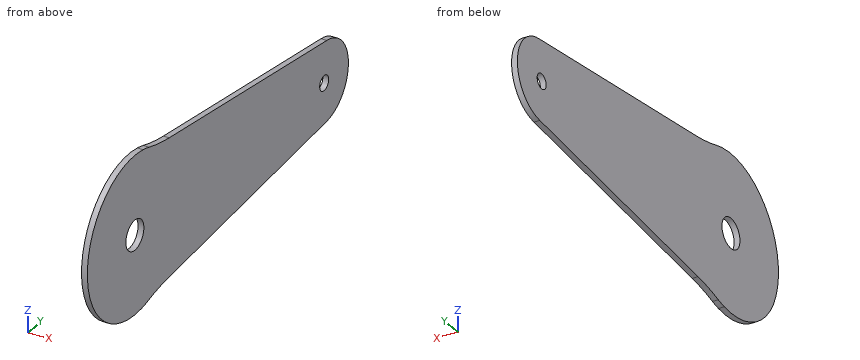
from build123d import *

# Parameters (mm, degrees)
SKETCH_2_R      = 3.85
SKETCH_2_R_2    = 1.925
EXTRUDE_1_DEPTH = 1.5


with BuildPart() as part:
    # 草圖2 → 填料-伸長1 (new body)
    with BuildSketch(Plane(origin=(0, 0, 0), x_dir=(0, 0, -1), z_dir=(1, 0, 0))):
        with BuildLine():
            Line((18.012072511, -21.441606673), (11.718522882, 46.276737912))
            ThreePointArc((11.718522882, 46.276737912), (1.55399875, 55.843411078), (-8.930005845, 46.627965677))
            Line((-8.930005845, 46.627965677), (-17.523002046, -20.837161438))
            ThreePointArc((-17.523002046, -20.837161438), (-18.27264724, -25.183298229), (-19.402359762, -29.446468708))
            ThreePointArc((-19.402359762, -29.446468708), (-19.752456192, -30.70663404), (-20.020797275, -31.986703271))
            ThreePointArc((-20.020797275, -31.986703271), (-0.345749536, -55.841970902), (20.12922907, -32.669648007))
            ThreePointArc((20.12922907, -32.669648007), (19.904578122, -31.38119307), (19.597542195, -30.109850035))
            ThreePointArc((19.597542195, -30.109850035), (18.61347279, -25.810724505), (18.012072511, -21.441606673))
        make_face()
        with Locations((0, -35.515504866)):
            Circle(SKETCH_2_R, mode=Mode.SUBTRACT)
        with Locations((1.377596172, 45.472779649)):
            Circle(SKETCH_2_R_2, mode=Mode.SUBTRACT)
    extrude(amount=EXTRUDE_1_DEPTH)


solid = part.part
CAD build for the part. Positions are in the model's coordinates, mm. Round coordinates to 2 decimals unless told otherwise and drop trailing zeros. Write each loop counter-clockwise with the first axis right and the second up, starting at its lowest first coordinate (ties: lowest second). Pieces come first, ordered by that corner, then holes. Notation, with made-up numbers: M 31,14.5 L 41,14.5 A27 cw 41,44.5 Z; hole C 33,-27.5 d3. An arc over 180 degrees is marked long. Use a Markdown table: item, result. Add a question column.
1. Slice it at C-C on z = -7. Give the cut face in (x, y), then the cut area to 3 significant figures.
2. Slice it at B-B on y = 20. Give the cut face in (x, z).
3. Slice it at A-A on x = 0.4. Give the number of separate pieces and of enclosed holes in the cut face, then the cut area to 3 significant figures.
4. Drill centre lines: probe 1 along Y at (x, z) = (0.5, -1.5); probe 2 along Y at (x, z) = (0.7, 0); probe 3 along Z at (x, y) = (0.2, -38). Where is each one in solid material? Low to high.
Reply:
| question | item | result |
|---|---|---|
| 1 | outline | M 0,-54.6 L 1.5,-54.6 L 1.5,54.19 L 0,54.19 Z |
| 1 | area | 163 mm^2 |
| 2 | outline | M 0,-14.16 L 1.5,-14.16 L 1.5,12.32 L 0,12.32 Z |
| 3 | separate pieces | 1 |
| 3 | enclosed holes | 2 |
| 3 | area | 3,190 mm^2 |
| 4 | probe 1 | y = -55.79 to -39.06, -31.97 to 43.55, 47.39 to 55.84 |
| 4 | probe 2 | y = -55.84 to -39.37, -31.67 to 44.13, 46.82 to 55.75 |
| 4 | probe 3 | z = -20.18 to -2.94, 2.94 to 20.18 |
